from build123d import *

# Parameters (mm, degrees)
BOSS_EXTRUDE1_DEPTH = 381
FILLET1_R           = 0.889


with BuildPart() as part:
    # Sketch1 → Boss-Extrude1 (new body)
    with BuildSketch(Plane.XY):
        with BuildLine():
            Line((0, 0), (0, 6.35))
            ThreePointArc((0, 6.35), (-3.432615786, 8.609796095), (-4.7625, 12.498361062))
            Line((-4.7625, 12.498361062), (-4.7625, 36.5125))
            ThreePointArc((-4.7625, 36.5125), (-6.388490208, 38.099533318), (-7.935633548, 36.435542215))
            Line((-7.935633548, 36.435542215), (-7.2459333, 22.225))
            Line((-7.2459333, 22.225), (-7.9375, 20.121392457))
            Line((-7.9375, 20.121392457), (-7.092967191, 19.84375))
            Line((-7.092967191, 19.84375), (-6.401400491, 21.947357543))
            ThreePointArc((-6.401400491, 21.947357543), (-6.364969814, 22.105734183), (-6.357978513, 22.26809636))
            Line((-6.357978513, 22.26809636), (-7.047678761, 36.478638575))
            ThreePointArc((-7.047678761, 36.478638575), (-6.366935691, 37.21079466), (-5.6515, 36.5125))
            Line((-5.6515, 36.5125), (-5.6515, 12.498361062))
            ThreePointArc((-5.6515, 12.498361062), (-4.342529701, 8.346509818), (-0.889, 5.696150484))
            Line((-0.889, 5.696150484), (-0.889, 0))
            Line((-0.889, 0), (0, 0))
        make_face()
    extrude(amount=-BOSS_EXTRUDE1_DEPTH)

    # Fillet1
    fillet1_edges = [part.edges().sort_by_distance(p)[0] for p in [
        (0, 6.35, -190.5),
    ]]
    fillet(fillet1_edges, radius=FILLET1_R)


solid = part.part
Model file for the job. Use its own axes, mm. A direction names the side the tool comes from. Coordinates: 2 decimals unless noted, no trailing zeros. Order: outer loops, then holes, each group sorted by start corner. A loop starts at its lowest first (then second) coordinate and runs counter-clockwise, first axis right, second up. Notation, with made-up numbers: (45.5, 16) -> (70.5, 16) arc R20 cw to (70.5, 50) -> close; hole circle Ø3 at (-5, 46.25). An arc over 180 degrees is marked (long way). Return JSON: item names as keys, results as strings. Group by question number.
Item 1: Pull direction X, two halves, no side cores. Call faces 3 (the flat face through (-4.762, 24, -188)), 4 (the flat face through (-5, 22, -381)), 5 (the flat face through (-5.652, 25, -188)), 6 (the flat face through (-6.7, 29.3, -187.8)): pulls with the +X half, pulls with the -X half, needs draft (parallel to the pull), parting line crosses it, or undercut.
Item 2: Tool access for faces 1 (the flat face through (-7.596, 29.43, -187.833)), 2 (the cylindrical face through (-3.58, 8.81, -187.83)): list every direction of +Z, -Z, +X, -X, +Y, -Y with a clear straight run to the whole face (end or side of a thin tool).
Item 3: Saw through at A-A on y = 32. Write the cut outline in (x, z).
Item 4: Wall check: line 1 along X through (y, z) = (36.5, -328); line 2 along X through (y, z) = (12.5, -118); line 3 along X through (y, z) = (22.5, -107). Give the ranges that are in metal, low to high. Write a range as [from, to].
Item 5: Flat gauge pins, fed straight in: P1, Ø12, axis at y = 26.5, z = -305.5, coming from the -X side; P2, Ø4, axis at y = 24.5, z = -46, coming from the -X side; P3, Ø12, axis at y = 19.5, z = -241, coming from the +X side. Where does each tip first touch, or does it go through?
Values found:
{
 "1": {"face 3": "pulls with the +X half", "face 4": "needs draft", "face 5": "undercut", "face 6": "undercut"},
 "2": {"face 1": "+Z, -Z, -X", "face 2": "+Z, -Z, +X, +Y"},
 "3": {"outline": "(-7.72, -381) -> (-6.83, -381) -> (-6.83, 0) -> (-7.72, 0) -> close; (-5.65, -381) -> (-4.76, -381) -> (-4.76, 0) -> (-5.65, 0) -> close"},
 "4": {"line 1": "x = [-7.94, -7.05], [-5.65, -4.76]", "line 2": "x = [-5.65, -4.76]", "line 3": "x = [-7.26, -6.37], [-5.65, -4.76]"},
 "5": {"P1": "stops at x = -7.81", "P2": "stops at x = -7.45", "P3": "stops at x = -4.76"}
}
